```python
from build123d import *

# Parameters (mm, degrees)
BOSS_EXTRUDE1_DEPTH = 39.8
SKETCH2_R           = 1.85
CUT_EXTRUDE1_DEPTH  = 39.8
SKETCH3_R           = 5.975
CUT_EXTRUDE2_DEPTH  = 39.8
CHAMFER1_SIZE       = 10
FILLET1_R           = 3


with BuildPart() as part:
    # Sketch1 → Boss-Extrude1 (new body)
    with BuildSketch(Plane(origin=(0, 0, 0), x_dir=(1, 0, 0), z_dir=(0, 1, 0))):
        Polygon((0, 0), (0, 27.7), (3, 27.7), (3, 4), (15, 4), (15, 0), align=None)
    extrude(amount=BOSS_EXTRUDE1_DEPTH)

    # Sketch2 → Cut-Extrude1 (cut)
    with BuildSketch(Plane(origin=(0, 0, -4), x_dir=(-1, 0, 0), z_dir=(0, 0, -1))):
        with Locations((-9, 35.7)):
            Circle(SKETCH2_R)
        with Locations((-9, 4.1)):
            Circle(SKETCH2_R)
    extrude(amount=-CUT_EXTRUDE1_DEPTH, mode=Mode.SUBTRACT)

    # Sketch3 → Cut-Extrude2 (cut)
    with BuildSketch(Plane(origin=(3, 0, 0), x_dir=(0, 0, -1), z_dir=(1, 0, 0))):
        with Locations((15.85, 19.9)):
            Circle(SKETCH3_R)
    extrude(amount=-CUT_EXTRUDE2_DEPTH, mode=Mode.SUBTRACT)

    # Chamfer1
    chamfer1_edges = [part.edges().sort_by_distance(p)[0] for p in [
        (1.5, 39.8, -27.7),
        (1.5, 0, -27.7),
    ]]
    chamfer(chamfer1_edges, length=CHAMFER1_SIZE)

    # Fillet1
    fillet1_edges = [part.edges().sort_by_distance(p)[0] for p in [
        (3, 19.9, -4),
    ]]
    fillet(fillet1_edges, radius=FILLET1_R)


solid = part.part
```
Could you check a few things on this model? Use its own coordinates, in mm. A direction names the side the tool comes from. Round coordinates to 2 decimals unless told otherwise and drop trailing zeros. Write each loop counter-clockwise with the first axis right and the second up, starting at its lowest first coordinate (ties: lowest second). Pieces come first, ordered by that corner, then holes.
(1) For pin 1 (11 mm diameter, centred on y = 19.9, z = -15.85, fed in from +X); pin 2 (10.5 mm diameter, centred on y = 27.5, z = -18.5, fed in from +X), each with a flat end and sliding along its axis, tell me the tip position at first contact or that it passes through.
Findings below:
pin 1: passes through
pin 2: stops at x = 3
(2) Suppose I cut it at D-D on z = -2.5. Write out the boundary of the cut face in (x, y), and give its area (3 significant figures).
Findings below:
outline: (0, 0) - (15, 0) - (15, 39.8) - (0, 39.8) - close; hole circle Ø3.7 at (9, 4.1); hole circle Ø3.7 at (9, 35.7)
area: 575 mm2
(3) Suppose I cut it at B-B on z = -15.85. Write out the boundary of the cut face in (x, y) (3 decimals), and give its area (4 significant figures).
Findings below:
outline: (0, 0) - (3, 0) - (3, 13.925) - (0, 13.925) - close; (0, 25.875) - (3, 25.875) - (3, 39.8) - (0, 39.8) - close
area: 83.55 mm2
(4) Suppose I cut it at C-C on y = 12. Write out the boundary of the cut face in (x, z).
Findings below:
outline: (0, -27.7) - (3, -27.7) - (3, -7) arc R3 cw to (6, -4) - (15, -4) - (15, 0) - (0, 0) - close
(5) Which directions (+Z, -Z, +X, -X, +Y, -Y) give clear straight access to the entire face, cutting with the end or side of a thin tool? Please do faces 4 (the face through (8, 20, 0)), 5 (the face through (3, 20, -22)).
Findings below:
face 4: +Z, +X, -X, +Y, -Y
face 5: -Z, +X, +Y, -Y
(6) Thinking about a two-plate mould opening in Y: for faces 1 (the face through (8.146, 34.059, -2.028)), 2 (the face through (1.5, 34.7, -22.8)), 3 (the face through (1, 20, -27.7)), which applies, +Y half, -Y half, draft (parallel to the pull), parting line (faces both ways), or undercut?
Findings below:
face 1: undercut
face 2: +Y half
face 3: draft
(7) Suppose I cut it at A-A on y = 4.1. Write out the boundary of the cut face in (x, z), and give its area (3 significant figures).
Findings below:
outline: (0, -21.8) - (3, -21.8) - (3, -7) arc R3 cw to (6, -4) - (7.15, -4) - (7.15, 0) - (0, 0) - close; (10.85, -4) - (15, -4) - (15, 0) - (10.85, 0) - close
area: 101 mm2
(8) If I drill on probe 1 along Y at (x, z) = (1.85, -15.85) (3 decimals); probe 2 along Y at (x, z) = (9, -3.05); probe 3 along Y at (x, z) = (9.75, -2), over which ranges is the centre line in solid material (lowest first)?
Findings below:
probe 1: y = 0 to 13.925, 25.875 to 39.8
probe 2: y = 0 to 2.25, 5.95 to 33.85, 37.55 to 39.8
probe 3: y = 0 to 2.41, 5.79 to 34.01, 37.39 to 39.8
